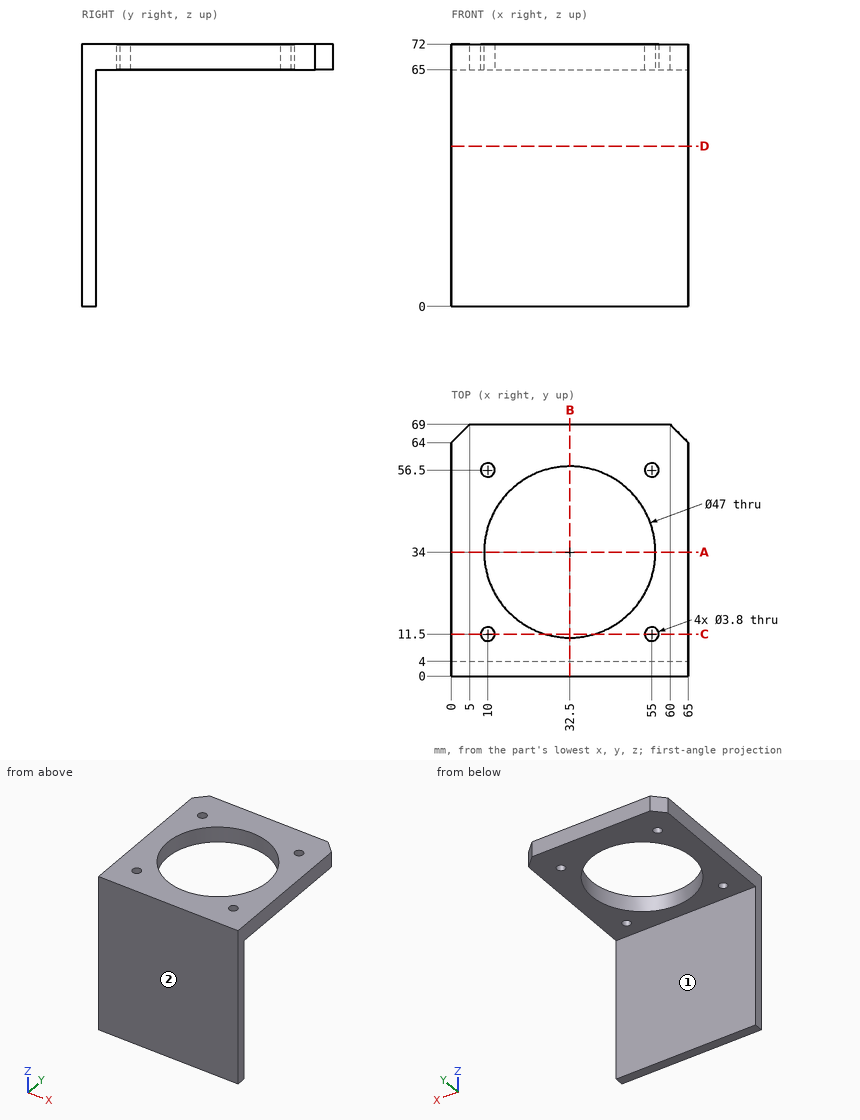
Job drawing, mm, ordinate dimensions from the low corner. One solid piece. A direction names the side the tool comes from. Coordinates: 2 decimals unless noted, no trailing zeros. Write each loop counter-clockwise with the first axis right and the second up, starting at its lowest first coordinate (ties: lowest second). Pieces come first, ordered by that corner, then holes. Notation, with made-up numbers: M 36.5,82.25 L 57.5,82.25 A29 ccw 57.5,109.25 Z; hole C 37,89 d5. An arc over 180 degrees is marked long. Answer as a JSON object with one key per item and string values. Group by question number.
1) Saw through at A-A (y = 34). Write the cut outline in (x, z).
2) Saw through at B-B (x = 32.5). Write the cut outline in (y, z).
3) Wall check: line 1 (Y direction, x = 57, z = 36); line 2 (Z direction, x = 7.5, y = 8). Give the ranges that are in metal, low to high. Write a range as from..to.
4) Tool access for the marked faces 1 and 2: list every direction of +Z, -Z, +X, -X, +Y, -Y with a clear straight run to the whole face (end or side of a thin tool).
5) Pin check, flat tips, straight feed: pin 1 Ø1 at (x, y) = (30, 56.5) entering from +Z; pin 2 Ø6 at (x, y) = (10, 11.5) entering from -Z; pin 3 Ø19.5 at (x, z) = (37.5, 23) entering from +Y. Stop position of each tip, or through.
6) Saw through at D-D (z = 44). Write the cut outline in (x, y), plus the area to 3 significant figures.
7) Saw through at C-C (y = 11.5). Write the cut outline in (x, z), plus the area to 3 significant figures.
Values follow:
{
 "1": {"outline": "M 0,65 L 9,65 L 9,72 L 0,72 Z; M 56,65 L 65,65 L 65,72 L 56,72 Z"},
 "2": {"outline": "M 0,0 L 4,0 L 4,65 L 10.5,65 L 10.5,72 L 0,72 Z; M 57.5,65 L 69,65 L 69,72 L 57.5,72 Z"},
 "3": {"line 1": "y = 0..4", "line 2": "z = 65..72"},
 "4": {"face 1": "-Z, +X, -X, +Y", "face 2": "+Z, -Z, +X, -X, -Y"},
 "5": {"pin 1": "passes through", "pin 2": "stops at z = 65", "pin 3": "stops at y = 4"},
 "6": {"outline": "M 0,0 L 65,0 L 65,4 L 0,4 Z", "area": "260 mm2"},
 "7": {"outline": "M 0,65 L 8.1,65 L 8.1,72 L 0,72 Z; M 11.9,65 L 25.72,65 L 25.72,72 L 11.9,72 Z; M 39.28,65 L 53.1,65 L 53.1,72 L 39.28,72 Z; M 56.9,65 L 65,65 L 65,72 L 56.9,72 Z", "area": "307 mm2"}
}
